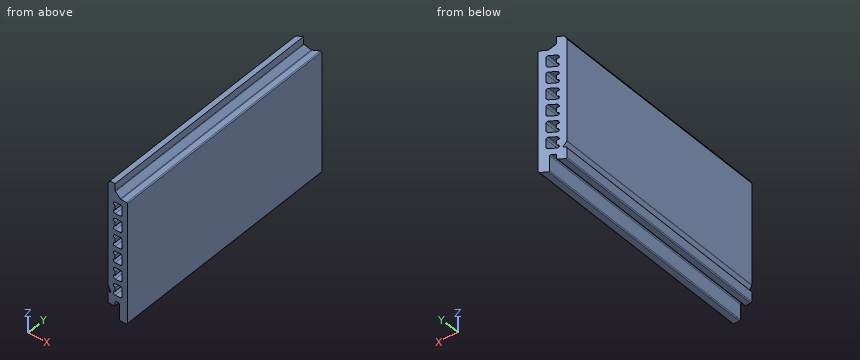
from build123d import *

# Parameters (mm, degrees)
F1_DEPTH      = 381
F3_DEPTH      = 711.2
F5_DEPTH      = 106.0997464
F5_DEPTH_BACK = 106.0997464


# Not quite as in the source:
# - ends of sketch curves that miss each other by under 0.0002 mm in the source are joined


with BuildPart() as f1:
    # F0 (on Front) → F1 (new body)
    with BuildSketch(Plane.XZ):
        with BuildLine():
            ThreePointArc((-14.9999680608, -58.9985104), (-14.96444377, -59.322873513), (-14.8595551032, -59.6318585804))
            Line((-14.8595551032, -59.6318585804), (-11.0988328608, -67.6967912))
            ThreePointArc((-11.0988328608, -67.6967912), (-11.1617050028, -68.655791158), (-12.004294, -69.1180454046))
            Line((-12.004294, -69.1180454046), (-14.0009118, -69.1180736))
            ThreePointArc((-14.0009118, -69.1180736), (-14.707352628, -69.410690972), (-14.99997, -70.1171318))
            Line((-14.99997, -70.1171318), (-14.99997, -85.599397))
            ThreePointArc((-14.99997, -85.599397), (-14.5606310505, -86.6600550505), (-13.499973, -87.099394))
            Line((-13.499973, -87.099394), (-5.5003446, -87.099394))
            ThreePointArc((-5.5003446, -87.099394), (-4.4396865495, -86.6600550505), (-4.0003476, -85.599397))
            Line((-4.0003476, -85.599397), (-4.0003476, -80.5996356))
            ThreePointArc((-4.0003476, -80.5996356), (-3.5610086505, -79.5389775495), (-2.5003506, -79.0996386))
            Line((-2.5003506, -79.0996386), (1.4838426, -79.0996386))
            ThreePointArc((1.4838426, -79.0996386), (2.5445365709, -79.5390134712), (2.9838395966, -80.5997372))
            Line((2.9838395966, -80.5997372), (2.98196, -104.5986224))
            ThreePointArc((2.98196, -104.5986224), (3.4212540492, -105.6593625482), (4.481957, -106.0987464))
            Line((4.481957, -106.0987464), (13.499973, -106.0987464))
            ThreePointArc((13.499973, -106.0987464), (14.5606310505, -105.6594074505), (14.99997, -104.5987494))
            Line((14.99997, -104.5987494), (14.99997, 83.7761342))
            ThreePointArc((14.99997, 83.7761342), (14.5844487053, 84.8124273268), (13.5680958768, 85.2745834897))
            Line((13.5680958768, 85.2745834897), (5.104384, 85.6592902))
            ThreePointArc((5.104384, 85.6592902), (4.5671403109, 85.7853117853), (4.1118233495, 86.0970797495))
            Line((4.1118233495, 86.0970797495), (-3.5610038, 93.7699166))
            ThreePointArc((-3.5610038, 93.7699166), (-3.8861671271, 94.2565457995), (-4.0003476, 94.8305698))
            Line((-4.0003476, 94.8305698), (-4.0003476, 106.0987464))
            Line((-4.0003476, 106.0987464), (-12.3105164, 106.0987464))
            Line((-12.3105164, 106.0987464), (-14.99997, 101.2086876))
            Line((-14.99997, 101.2086876), (-14.9999680608, -58.9985104))
        make_face()
    extrude(amount=F1_DEPTH)

    # F2 (on Front) → F3 (cut)
    with BuildSketch(Plane.XZ):
        with BuildLine():
            ThreePointArc((-5.49529, -31.195264), (-4.4346319495, -31.6346029495), (-3.995293, -32.695261))
            Line((-3.995293, -32.695261), (-3.995293, -37.695251))
            ThreePointArc((-3.995293, -37.695251), (-4.4346319495, -38.7559090505), (-5.49529, -39.195248))
            Line((-5.49529, -39.195248), (-5.499989, -39.195248))
            ThreePointArc((-5.499989, -39.195248), (-6.5606470505, -39.6345869495), (-6.999986, -40.695245))
            Line((-6.999986, -40.695245), (-6.999986, -41.195244))
            ThreePointArc((-6.999986, -41.195244), (-6.1213081009, -43.3165601009), (-3.999992, -44.195238))
            Line((-3.999992, -44.195238), (3.999992, -44.195238))
            ThreePointArc((3.999992, -44.195238), (6.1213081009, -43.3165601009), (6.999986, -41.195244))
            Line((6.999986, -41.195244), (6.999986, -29.195268))
            ThreePointArc((6.999986, -29.195268), (6.1213081009, -27.0739518991), (3.999992, -26.195274))
            Line((3.999992, -26.195274), (-3.999992, -26.195274))
            ThreePointArc((-3.999992, -26.195274), (-6.1213081009, -27.0739518991), (-6.999986, -29.195268))
            Line((-6.999986, -29.195268), (-6.999986, -29.695267))
            ThreePointArc((-6.999986, -29.695267), (-6.5606470505, -30.7559250505), (-5.499989, -31.195264))
            Line((-5.499989, -31.195264), (-5.49529, -31.195264))
        make_face()
        with BuildLine():
            ThreePointArc((-5.49529, -56.595264), (-4.4346319495, -57.0346029495), (-3.995293, -58.095261))
            Line((-3.995293, -58.095261), (-3.995293, -63.095251))
            ThreePointArc((-3.995293, -63.095251), (-4.4346319495, -64.1559090505), (-5.49529, -64.595248))
            Line((-5.49529, -64.595248), (-5.499989, -64.595248))
            ThreePointArc((-5.499989, -64.595248), (-6.5606470505, -65.0345869495), (-6.999986, -66.095245))
            Line((-6.999986, -66.095245), (-6.999986, -66.595244))
            ThreePointArc((-6.999986, -66.595244), (-6.1213081009, -68.7165601009), (-3.999992, -69.595238))
            Line((-3.999992, -69.595238), (0, -69.595238))
            Line((0, -69.595238), (3.999992, -69.595238))
            ThreePointArc((3.999992, -69.595238), (6.1213081009, -68.7165601009), (6.999986, -66.595244))
            Line((6.999986, -66.595244), (6.999986, -54.595268))
            ThreePointArc((6.999986, -54.595268), (6.1213081009, -52.4739518991), (3.999992, -51.595274))
            Line((3.999992, -51.595274), (-3.999992, -51.595274))
            ThreePointArc((-3.999992, -51.595274), (-6.1213081009, -52.4739518991), (-6.999986, -54.595268))
            Line((-6.999986, -54.595268), (-6.999986, -55.095267))
            ThreePointArc((-6.999986, -55.095267), (-6.5606470505, -56.1559250505), (-5.499989, -56.595264))
            Line((-5.499989, -56.595264), (-5.49529, -56.595264))
        make_face()
        with BuildLine():
            ThreePointArc((-5.49529, -5.3953664), (-4.4346319495, -5.8347053495), (-3.995293, -6.8953634))
            Line((-3.995293, -6.8953634), (-3.995293, -11.8953534))
            ThreePointArc((-3.995293, -11.8953534), (-4.4346319495, -12.9560114505), (-5.49529, -13.3953504))
            Line((-5.49529, -13.3953504), (-5.499989, -13.3953504))
            ThreePointArc((-5.499989, -13.3953504), (-6.5606470505, -13.8346893495), (-6.999986, -14.8953474))
            Line((-6.999986, -14.8953474), (-6.999986, -15.3953464))
            ThreePointArc((-6.999986, -15.3953464), (-6.1213081009, -17.5166625009), (-3.999992, -18.3953404))
            Line((-3.999992, -18.3953404), (3.999992, -18.3953404))
            ThreePointArc((3.999992, -18.3953404), (6.1213081009, -17.5166625009), (6.999986, -15.3953464))
            Line((6.999986, -15.3953464), (6.999986, -3.3953704))
            ThreePointArc((6.999986, -3.3953704), (6.1213081009, -1.2740542991), (3.999992, -0.3953764))
            Line((3.999992, -0.3953764), (-3.999992, -0.3953764))
            ThreePointArc((-3.999992, -0.3953764), (-6.1213081009, -1.2740542991), (-6.999986, -3.3953704))
            Line((-6.999986, -3.3953704), (-6.999986, -3.8953694))
            ThreePointArc((-6.999986, -3.8953694), (-6.5606470505, -4.9560274505), (-5.499989, -5.3953664))
            Line((-5.499989, -5.3953664), (-5.49529, -5.3953664))
        make_face()
        with BuildLine():
            Line((-5.499989, 20.4015086), (-5.49529, 20.4015086))
            ThreePointArc((-5.49529, 20.4015086), (-4.4346319495, 19.9621696505), (-3.995293, 18.9015116))
            Line((-3.995293, 18.9015116), (-3.995293, 13.9015216))
            ThreePointArc((-3.995293, 13.9015216), (-4.4346319495, 12.8408635495), (-5.49529, 12.4015246))
            Line((-5.49529, 12.4015246), (-5.499989, 12.4015246))
            ThreePointArc((-5.499989, 12.4015246), (-6.5606470505, 11.9621856505), (-6.999986, 10.9015276))
            Line((-6.999986, 10.9015276), (-6.999986, 10.4015286))
            ThreePointArc((-6.999986, 10.4015286), (-6.1213081009, 8.2802124991), (-3.999992, 7.4015346))
            Line((-3.999992, 7.4015346), (3.999992, 7.4015346))
            ThreePointArc((3.999992, 7.4015346), (6.1213081009, 8.2802124991), (6.999986, 10.4015286))
            Line((6.999986, 10.4015286), (6.999986, 22.4015046))
            ThreePointArc((6.999986, 22.4015046), (6.1213081009, 24.5228207009), (3.999992, 25.4014986))
            Line((3.999992, 25.4014986), (-3.999992, 25.4014986))
            ThreePointArc((-3.999992, 25.4014986), (-6.1213081009, 24.5228207009), (-6.999986, 22.4015046))
            Line((-6.999986, 22.4015046), (-6.999986, 21.9015056))
            ThreePointArc((-6.999986, 21.9015056), (-6.5606470505, 20.8408475495), (-5.499989, 20.4015086))
        make_face()
        with BuildLine():
            Line((-5.499989, 46.1983836), (-5.49529, 46.1983836))
            ThreePointArc((-5.49529, 46.1983836), (-4.4346319495, 45.7590446505), (-3.995293, 44.6983866))
            Line((-3.995293, 44.6983866), (-3.995293, 39.6983966))
            ThreePointArc((-3.995293, 39.6983966), (-4.4346319495, 38.6377385495), (-5.49529, 38.1983996))
            Line((-5.49529, 38.1983996), (-5.499989, 38.1983996))
            ThreePointArc((-5.499989, 38.1983996), (-6.5606470505, 37.7590606505), (-6.999986, 36.6984026))
            Line((-6.999986, 36.6984026), (-6.999986, 36.1984036))
            ThreePointArc((-6.999986, 36.1984036), (-6.1213081009, 34.0770874991), (-3.999992, 33.1984096))
            Line((-3.999992, 33.1984096), (3.999992, 33.1984096))
            ThreePointArc((3.999992, 33.1984096), (6.1213081009, 34.0770874991), (6.999986, 36.1984036))
            Line((6.999986, 36.1984036), (6.999986, 48.1983796))
            ThreePointArc((6.999986, 48.1983796), (6.1213081009, 50.3196957009), (3.999992, 51.1983736))
            Line((3.999992, 51.1983736), (-3.999992, 51.1983736))
            ThreePointArc((-3.999992, 51.1983736), (-6.1213081009, 50.3196957009), (-6.999986, 48.1983796))
            Line((-6.999986, 48.1983796), (-6.999986, 47.6983806))
            ThreePointArc((-6.999986, 47.6983806), (-6.5606470505, 46.6377225495), (-5.499989, 46.1983836))
        make_face()
        with BuildLine():
            Line((-5.499989, 71.9952586), (-5.49529, 71.9952586))
            ThreePointArc((-5.49529, 71.9952586), (-4.4346319495, 71.5559196505), (-3.995293, 70.4952616))
            Line((-3.995293, 70.4952616), (-3.995293, 65.4952716))
            ThreePointArc((-3.995293, 65.4952716), (-4.4346319495, 64.4346135495), (-5.49529, 63.9952746))
            Line((-5.49529, 63.9952746), (-5.499989, 63.9952746))
            ThreePointArc((-5.499989, 63.9952746), (-6.5606470505, 63.5559356505), (-6.999986, 62.4952776))
            Line((-6.999986, 62.4952776), (-6.999986, 61.9952786))
            ThreePointArc((-6.999986, 61.9952786), (-6.1213081009, 59.8739624991), (-3.999992, 58.9952846))
            Line((-3.999992, 58.9952846), (3.999992, 58.9952846))
            ThreePointArc((3.999992, 58.9952846), (6.1213081009, 59.8739624991), (6.999986, 61.9952786))
            Line((6.999986, 61.9952786), (6.999986, 73.9952546))
            ThreePointArc((6.999986, 73.9952546), (6.1213081009, 76.1165707009), (3.999992, 76.9952486))
            Line((3.999992, 76.9952486), (-3.999992, 76.9952486))
            ThreePointArc((-3.999992, 76.9952486), (-6.1213081009, 76.1165707009), (-6.999986, 73.9952546))
            Line((-6.999986, 73.9952546), (-6.999986, 73.4952556))
            ThreePointArc((-6.999986, 73.4952556), (-6.5606470505, 72.4345975495), (-5.499989, 71.9952586))
        make_face()
    extrude(amount=F3_DEPTH, mode=Mode.SUBTRACT)

    # F4 (on Top) → F5 (cut, two sides)
    with BuildSketch(Plane.XY) as f5_sk:
        Polygon((15.1597065851, 0), (-15.0980791077, 0), (-15.0980791077, -19.05), align=None)
    extrude(amount=-F5_DEPTH, mode=Mode.SUBTRACT)
    extrude(f5_sk.sketch, amount=F5_DEPTH_BACK, mode=Mode.SUBTRACT)


solid = f1.part
Read the model definition and answer for the solid it produces. Units are mm, in the model's axes. Coordinates: 2 decimals unless noted, no trailing zeros. Answer in a Markdown table with one row per item.
Q1. Given P1, Ø4, axis at x = -1, y = -231, coming from the +Z side; P2, Ø3, axis at x = 10, z = 17, coming from the +Y side; P3, Ø8, axis at x = -3.5, y = -291, coming from the +Z side; P4, Ø9, axis at y = -135.5, z = 99.5, coming from the +X side, each flat-ended and moving along its own axis, determine where each tip first touches the part or whether it passes through.
Here are the results:
| item | result |
|---|---|
| P1 | stops at z = 93.21 |
| P2 | stops at y = -2.3 |
| P3 | stops at z = 106.1 |
| P4 | stops at x = -4 |
Q2. Find section A-A on y = -91. Count the separate pieces of the cut face and the enclosed holes in it, plus the area to 3 significant figures.
Here are the results:
| item | result |
|---|---|
| separate pieces | 1 |
| enclosed holes | 6 |
| area | 4,260 mm^2 |
Q3. Straight lines are drawn through the part: line 1 along X through (y, z) = (-267.5, 48); line 2 along X through (y, z) = (-80, -32); line 3 along Y through (x, z) = (13.5, 37.5). For each, find the intervals that lie inside material, in ascending order. Write a range as [from, to].
Here are the results:
| item | result |
|---|---|
| line 1 | x = [-15, -7], [7, 15] |
| line 2 | x = [-15, -4.17], [7, 15] |
| line 3 | y = [-381, -1.04] |
